Here's how the part is built. I have some questions about the finished solid (model axes, mm). Round coordinates to 2 decimals unless told otherwise and drop trailing zeros. Loops run counter-clockwise (first coordinate to the right, second up) from the corner with the lowest first, then second, coordinate; pieces in that order, holes last. Notation, with made-up numbers: (-34, 86) -> (-15, 86) arc R23 cw to (-15, 101) -> close; hole circle Ø7 at (47, 10.5). An arc over 180 degrees is marked (long way). Use one line per item in the form item = value. Start each with the question number.
Item 1: If we section it at B-B (x = 0.5): Write out the boundary of the cut face in (y, z).
Item 2: I'm going to push flat-ended pins straight in: pin 1 Ø1.2 at (y, z) = (8, 1.5) entering from +X; pin 2 Ø1 at (x, z) = (21, 0.5) entering from -Y. Where does each tip first touch, or does it pass through?
Item 3: If we section it at D-D (x = 18.5): Write out the boundary of the cut face in (y, z), then the cut area to 3 significant figures.
Item 4: If we section it at C-C (y = -36.5): Write out the boundary of the cut face in (x, z).
Item 5: If we section it at A-A (x = -13.5): Write out the boundary of the cut face in (y, z), then the cut area to 3 significant figures.
Item 6: Thinking about a two-plate mould opening in Y: for faces 1 (the face through (22, 37.2, 2)), 2 (the face through (27.5, -1, 1)), 3 (the face through (16.6, 12, 2)), 4 (the face through (0, -40.7, 1)), which applies, released by +Y, released by -Y, zero draft, split by the parting line, or undercut?
Item 7: If I drill on L1, parallel to Y at x = 11, z = 1.5; L2, parallel to X at y = -22, z = 0.55; L3, parallel to Y at x = -15.5, z = 0.8, over which ranges is the centre line in solid material (lowest first)? Write a range as [from, to].
```python
from build123d import *

# Parameters (mm, degrees)
SKETCH_W      = 55
SKETCH_H      = 81.4
SKETCH_W_2    = 4
SKETCH_H_2    = 50
SKETCH_H_3    = 35
SKETCH_W_3    = 3.15
SKETCH_H_4    = 13.3
SKETCH_W_4    = 13.42
SKETCH_H_5    = 15.1
SKETCH_W_5    = 40
SKETCH_H_6    = 3.5
PAD_DEPTH     = 4
SKETCH001_W   = 61
SKETCH001_H   = 87.4
SKETCH001_W_2 = 55
SKETCH001_H_2 = 81.4
PAD001_DEPTH  = 1.5


with BuildPart() as part:
    # Sketch → Pad (new body)
    with BuildSketch(Plane.XY):
        Rectangle(SKETCH_W, SKETCH_H)
        with Locations((-21.9, 12.2)):
            Rectangle(SKETCH_W_2, SKETCH_H_2, mode=Mode.SUBTRACT)
        with Locations((-14.6, 12.2)):
            Rectangle(SKETCH_W_2, SKETCH_H_2, mode=Mode.SUBTRACT)
        with Locations((-7.3, 12.2)):
            Rectangle(SKETCH_W_2, SKETCH_H_2, mode=Mode.SUBTRACT)
        with Locations((0, 12.2)):
            Rectangle(SKETCH_W_2, SKETCH_H_2, mode=Mode.SUBTRACT)
        with Locations((7.3, 12.2)):
            Rectangle(SKETCH_W_2, SKETCH_H_2, mode=Mode.SUBTRACT)
        with Locations((14.6, 12.2)):
            Rectangle(SKETCH_W_2, SKETCH_H_2, mode=Mode.SUBTRACT)
        with Locations((21.9, 19.7)):
            Rectangle(SKETCH_W_2, SKETCH_H_3, mode=Mode.SUBTRACT)
        with Locations((21.475, -6.15)):
            Rectangle(SKETCH_W_3, SKETCH_H_4, mode=Mode.SUBTRACT)
        with Locations((-10.71, -22.35)):
            Rectangle(SKETCH_W_4, SKETCH_H_5, mode=Mode.SUBTRACT)
        with Locations((9.99, -22.35)):
            Rectangle(SKETCH_W_4, SKETCH_H_5, mode=Mode.SUBTRACT)
        with Locations((0, -36.45)):
            Rectangle(SKETCH_W_5, SKETCH_H_6, mode=Mode.SUBTRACT)
    extrude(amount=PAD_DEPTH)

    # Sketch001 → Pad001 (new body)
    with BuildSketch(Plane.XY.offset(4)):
        Rectangle(SKETCH001_W, SKETCH001_H)
        Rectangle(SKETCH001_W_2, SKETCH001_H_2, mode=Mode.SUBTRACT)
    extrude(amount=-PAD001_DEPTH)


solid = part.part
```
Values found:
q1.outline = (-43.7, 2.5) -> (-40.7, 2.5) -> (-40.7, 0) -> (-38.2, 0) -> (-38.2, 4) -> (-43.7, 4) -> close; (-34.7, 0) -> (-12.8, 0) -> (-12.8, 4) -> (-34.7, 4) -> close; (37.2, 0) -> (40.7, 0) -> (40.7, 2.5) -> (43.7, 2.5) -> (43.7, 4) -> (37.2, 4) -> close
q2.pin_1 = 27.5
q2.pin_2 = -40.7
q3.outline = (-43.7, 2.5) -> (-40.7, 2.5) -> (-40.7, 0) -> (-38.2, 0) -> (-38.2, 4) -> (-43.7, 4) -> close; (-34.7, 0) -> (40.7, 0) -> (40.7, 2.5) -> (43.7, 2.5) -> (43.7, 4) -> (-34.7, 4) -> close
q3.area = 321 mm2
q4.outline = (-30.5, 2.5) -> (-27.5, 2.5) -> (-27.5, 0) -> (-20, 0) -> (-20, 4) -> (-30.5, 4) -> close; (20, 0) -> (27.5, 0) -> (27.5, 2.5) -> (30.5, 2.5) -> (30.5, 4) -> (20, 4) -> close
q5.outline = (-43.7, 2.5) -> (-40.7, 2.5) -> (-40.7, 0) -> (-38.2, 0) -> (-38.2, 4) -> (-43.7, 4) -> close; (-34.7, 0) -> (-29.9, 0) -> (-29.9, 4) -> (-34.7, 4) -> close; (-14.8, 0) -> (-12.8, 0) -> (-12.8, 4) -> (-14.8, 4) -> close; (37.2, 0) -> (40.7, 0) -> (40.7, 2.5) -> (43.7, 2.5) -> (43.7, 4) -> (37.2, 4) -> close
q5.area = 60.2 mm2
q6.face_1 = undercut
q6.face_2 = zero draft
q6.face_3 = undercut
q6.face_4 = released by -Y
q7.L1 = [-40.7, -38.2], [-34.7, -29.9], [-14.8, 40.7]
q7.L2 = [-27.5, -17.42], [-4, 3.28], [16.7, 27.5]
q7.L3 = [-40.7, -38.2], [-34.7, -29.9], [-14.8, -12.8], [37.2, 40.7]
